from build123d import *

# Parameters (mm, degrees)
F0_W     = 517
F0_H     = 437.351066
F1_DEPTH = 480
F2_T     = -2.5
F3_R     = 5
F5_R     = 15
F5_R_2   = 12.5
F6_DEPTH = 11.75
F7_R     = 3
F8_DEPTH = 12.5


with BuildPart() as f1:
    # F0 (on Top) → F1 (new body)
    with BuildSketch(Plane.XY):
        with Locations((154.318035, -9.831567)):
            Rectangle(F0_W, F0_H)
    extrude(amount=F1_DEPTH)

    # F2
    f2_openings = [f1.faces().sort_by_distance(p)[0] for p in [
        (154.318035, -228.5071, 240),
        (154.318035, -9.831567, 0),
    ]]
    offset(amount=F2_T, openings=f2_openings)

    # F3
    f3_edges = [f1.edges().sort_by_distance(p)[0] for p in [
        (412.818035, -9.831567, 480),
        (-104.181965, -9.831567, 480),
        (412.818035, 208.843966, 240),
        (154.318035, 208.843966, 480),
        (-104.181965, 208.843966, 240),
    ]]
    fillet(f3_edges, radius=F3_R)

    # F5 (on face) → F6 (cut)
    with BuildSketch(Plane(origin=(0, 208.843966, 0), x_dir=(-1, 0, 0), z_dir=(0, 1, 0))):
        with Locations((-364.1496, 30.58356)):
            Circle(F5_R)
        with Locations((38.893182, 35.777409)):
            Circle(F5_R_2)
    extrude(amount=-F6_DEPTH, mode=Mode.SUBTRACT)

    # F7 (on face) → F8 (cut)
    with BuildSketch(Plane.XY.offset(480)):
        with Locations((154.318035, -12.331567)):
            Circle(F7_R)
    extrude(amount=-F8_DEPTH, mode=Mode.SUBTRACT)


solid = f1.part
Read the model definition and answer for the solid it produces. Units are mm, in the model's axes. A direction names the side the tool comes from. Round coordinates to 2 decimals unless told otherwise and drop trailing zeros. Write each loop counter-clockwise with the first axis right and the second up, starting at its lowest first coordinate (ties: lowest second). Pieces come first, ordered by that corner, then holes.
Q1. Find section C-C on z = 211. Determine the outline of the cut face in (x, y), and give its area (3 significant figures).
Values:
outline: (-104.18, -228.51) - (-101.68, -228.51) - (-101.68, 206.34) - (410.32, 206.34) - (410.32, -228.51) - (412.82, -228.51) - (412.82, 203.84) arc R5 ccw to (407.82, 208.84) - (-99.18, 208.84) arc R5 ccw to (-104.18, 203.84) - close
area: 3,460 mm2
Q2. Find section A-A on y = 113.5. Determine the outline of the cut face in (x, z).
Values:
outline: (-104.18, 0) - (-101.68, 0) - (-101.68, 477.5) - (410.32, 477.5) - (410.32, 0) - (412.82, 0) - (412.82, 475) arc R5 ccw to (407.82, 480) - (-99.18, 480) arc R5 ccw to (-104.18, 475) - close
Q3. Straight lines are drawn through the part: line 1 (X direction, y = 114, z = 228); line 2 (Y direction, x = 213, z = 407.5); line 3 (Z direction, x = 177, y = -35). For each, find the intervals that lie inside material, in ascending order.
Values:
line 1: x = -104.18 to -101.68, 410.32 to 412.82
line 2: y = 206.34 to 208.84
line 3: z = 477.5 to 480
Q4. The mould has two halves that part along Z. Classify faces 1 (the face through (151, -9, 480)), 2 (the face through (356.086, 207.611, 43.232)), 3 (the face through (412.818, -15, 234)), 4 (the face through (-45.61, 207.61, 46.32)): released by +Z, released by -Z, zero draft, split by the parting line, or undercut.
Values:
face 1: released by +Z
face 2: undercut
face 3: zero draft
face 4: undercut
Q5. Flat-ended cylindrical pins translate along their axes: P1, Ø3, axis at x = 223, y = -40.5, coming from the -Z side; P2, Ø22.5, axis at x = -38.89, z = 35.78, coming from the -Y side; P3, Ø10, axis at x = 337, z = 205, coming from the -Y side. Find the tip coordinate at first contact, or state that the pin passes through.
Values:
P1: stops at z = 477.5
P2: passes through
P3: stops at y = 206.34
Q6. A tool of negligible diameter and unlimited length cuts with its end or side. For faces 5 (the face through (151, -8, 477.5)), 6 (the face through (151, 208.844, 234)), from which of +Z, -Z, +X, -X, +Y, -Y can it reach the whole face along a straight path? Write none if from no direction.
Values:
face 5: -Z, -Y
face 6: +Z, -Z, +X, -X, +Y
Q7. Find section B-B on x = 357.5. Determine the outline of the cut face in (y, z), and give its area (3 significant figures).
Values:
outline: (-228.51, 477.5) - (206.34, 477.5) - (206.34, 44.03) - (208.84, 44.03) - (208.84, 475) arc R5 ccw to (203.84, 480) - (-228.51, 480) - close; (206.34, 0) - (208.84, 0) - (208.84, 17.14) - (206.34, 17.14) - close
area: 2,210 mm2
